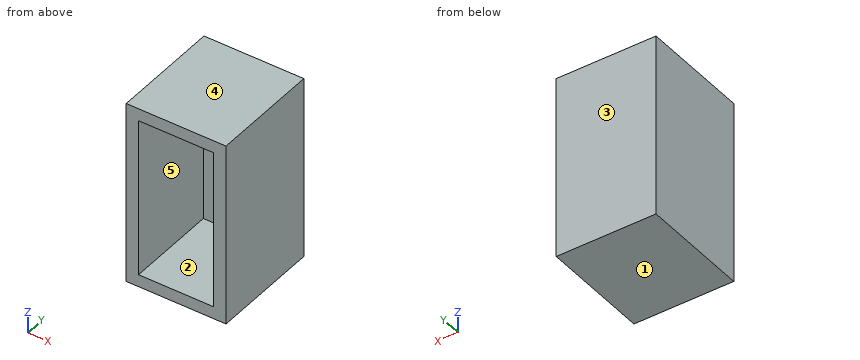
Autodesk Fusion 360 part; units mm, degrees
sketch "Sketch1" plane through (0, 0, 0) normal (0, 1, 0) x (1, 0, 0)
  line L0 (0, 0) -> (16.2, 0)
  line L1 (16.2, 0) -> (16.2, -29.8)
  line L2 (16.2, -29.8) -> (0, -29.8)
  line L3 (0, -29.8) -> (0, 0)
  dimension "d1" = 16.2
  dimension "d2" = 29.8
extrude "Extrude1" add sketch "Sketch1" along normal blind 18
sketch "Sketch2" plane through (0, 0, 0) normal (0, -1, 0) x (1, 0, 0)
  line L0 (16.2, 29.8) -> (0, 29.8)
  line L1 (0, 29.8) -> (0, 0)
  line L2 (0, 0) -> (16.2, 0)
  line L3 (16.2, 0) -> (16.2, 29.8)
  line L4 (0, 29.8) -> (2, 29.8)
  line L5 (2, 29.8) -> (2, 27.8)
  line L6 (2, 27.8) -> (14.2, 27.8)
  line L7 (14.2, 27.8) -> (14.2, 2)
  line L8 (14.2, 2) -> (2, 2)
  line L9 (2, 2) -> (2, 27.8)
  dimension "d5" = 2
  dimension "d6" = 2
  dimension "d7" = 12.2
  dimension "d8" = 25.8
extrude "Extrude2" cut sketch "Sketch2" against normal blind 15 contours L6 L7 L8 L9
Check sheet for the modelled part. Datum: model origin and axes. Units: mm. Face numbers are marked on the shaded views. A direction names the side the tool comes from. Give positions to 0.01 mm unless a question says otherwise; leave off trailing zeros. Order: outer loops, then holes, each group sorted by start corner. A loop starts at its lowest first (then second) coordinate and runs counter-clockwise, first axis right, second up. Notation, with made-up numbers: (-30, 29.25) -> (11, 29.25) arc R17 ccw to (11, 39.25) -> close; hole circle Ø2 at (-37.75, -26.75). An arc over 180 degrees is marked (long way). Return JSON: item names as keys, results as strings.
1. Cross-section at B-B, the plane y = 13. Record the cut outline in (x, z), plus the area to 3 significant figures.
From the geometry:
{"outline": "(0, 0) -> (16.2, 0) -> (16.2, 29.8) -> (0, 29.8) -> close; hole (2, 2) -> (14.2, 2) -> (14.2, 27.8) -> (2, 27.8) -> close", "area": "168 mm^2"}
2. Cross-section at C-C, the plane x = 10. Record the cut outline in (y, z).
From the geometry:
{"outline": "(0, 0) -> (18, 0) -> (18, 29.8) -> (0, 29.8) -> (0, 27.8) -> (15, 27.8) -> (15, 2) -> (0, 2) -> close"}
3. Mould release check, pull along Z, two halves, no side actions. Record for the marked faces 3, 4 and 5: +Z half, -Z half, draft (parallel to the pull), parting line (faces both ways), or undercut.
From the geometry:
{"face 3": "draft", "face 4": "+Z half", "face 5": "undercut"}
4. Material ranges on probe 1 along X at (y, z) = (8.5, 26); probe 2 along Z at (x, y) = (4.75, 3.5); probe 3 along Y at (x, z) = (3.5, 8), recorded low to high. Write a range as [from, to].
From the geometry:
{"probe 1": "[0, 2], [14.2, 16.2]", "probe 2": "[0, 2], [27.8, 29.8]", "probe 3": "[15, 18]"}
5. Set-up check for the marked faces 1 and 2: record each of +Z, -Z, +X, -X, +Y, -Y from which the full face is reachable in a straight line by a thin tool's end or side.
From the geometry:
{"face 1": "-Z, +X, -X, +Y, -Y", "face 2": "-Y"}
6. Go/stop test with flat-tipped pins: P1, Ø3, axis at x = 6.5, y = 2.5, coming from the -Z side; P2, Ø3.5, axis at x = 9, z = 10, coming from the -Y side. Record where each tip stops, or that it passes through.
From the geometry:
{"P1": "z = 0", "P2": "y = 15"}
7. Cross-section at A-A, the plane z = 4.75. Record the cut outline in (x, y), plus the area to 3 significant figures.
From the geometry:
{"outline": "(0, 0) -> (2, 0) -> (2, 15) -> (14.2, 15) -> (14.2, 0) -> (16.2, 0) -> (16.2, 18) -> (0, 18) -> close", "area": "109 mm^2"}
